Design review of the part shown in the three views and the two pictorial views. Dimensions are in mm from the part's minimum x, y and z. Give positions to 0.01 mm unless a question says otherwise; leave off trailing zeros. Loops run counter-clockwise (first coordinate to the right, second up) from the corner with the lowest first, then second, coordinate; pieces in that order, holes last. Notation, with made-up numbers: (78, 34.5) -> (136, 34.5) arc R16 cw to (136, 47.5) -> close; hole circle Ø10 at (-7, -15). An arc over 180 degrees is marked (long way). One line per question, with ' | ' between items. Start each with the question number.
(1) Consider section B-B (z = 44). Write out the cut boundary in (x, y).
(2) Insertion check: P1, Ø0.9, axis at y = 35.5, z = 79, coming from the +X side; P2, Ø1.5, axis at x = 71.5, z = 16.5, coming from the -Y side; P3, Ø1.5, axis at y = 16.5, z = 10.5, coming from the +X side. Each pin has a flat end and moves straight along its axis. Give the tip position at first contact, or say it passes through.
(3) Consider section A-A (x = 105). Write out the cut boundary in (y, z).
(4) Consider section D-D (x = 38). Write out the cut boundary in (y, z).
(5) Consider section C-C (y = 56). Write out the cut boundary in (x, z) (1 decimal).
(6) Wall thickness on probe 1 along X at (y, z) = (35, 51.5) (1 decimal); probe 2 along X at (y, z) = (56, 23.5) (1 decimal); probe 3 along Z at (x, y) = (63.5, 39.5): over which ranges is each line inside the solid? List them lowest first.
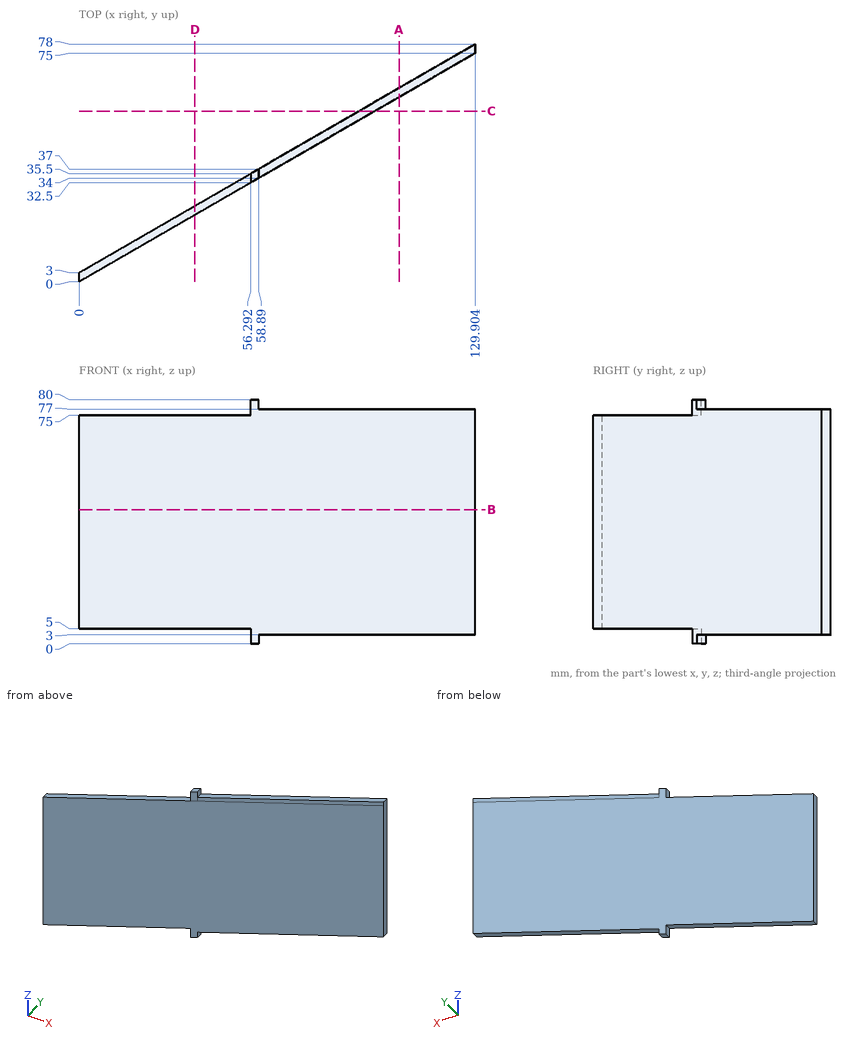
A:
1) outline: (0, 0) -> (129.9, 75) -> (129.9, 78) -> (0, 3) -> close
2) P1: stops at x = 58.89 | P2: stops at y = 40.85 | P3: stops at x = 29.88
3) outline: (60.62, 3) -> (63.62, 3) -> (63.62, 77) -> (60.62, 77) -> close
4) outline: (21.94, 5) -> (24.94, 5) -> (24.94, 75) -> (21.94, 75) -> close
5) outline: (91.8, 3) -> (97, 3) -> (97, 77) -> (91.8, 77) -> close
6) probe 1: x = 55.4 to 60.6 | probe 2: x = 91.8 to 97 | probe 3: z = 3 to 77
